Part print with two shaded views. Sizes in mm from the minimum x, y, z corner. Coordinates: 2 decimals unless noted, no trailing zeros. Order: outer loops, then holes, each group sorted by start corner. A loop starts at its lowest first (then second) coordinate and runs counter-clockwise, first axis right, second up. Notation, with made-up numbers: M -12,7 L 17,7 A12 ccw 17,21 Z; hole C 37.5,-20.5 d6. An arc over 180 degrees is marked long. Answer in a Markdown table with one row per item. Add a question column.
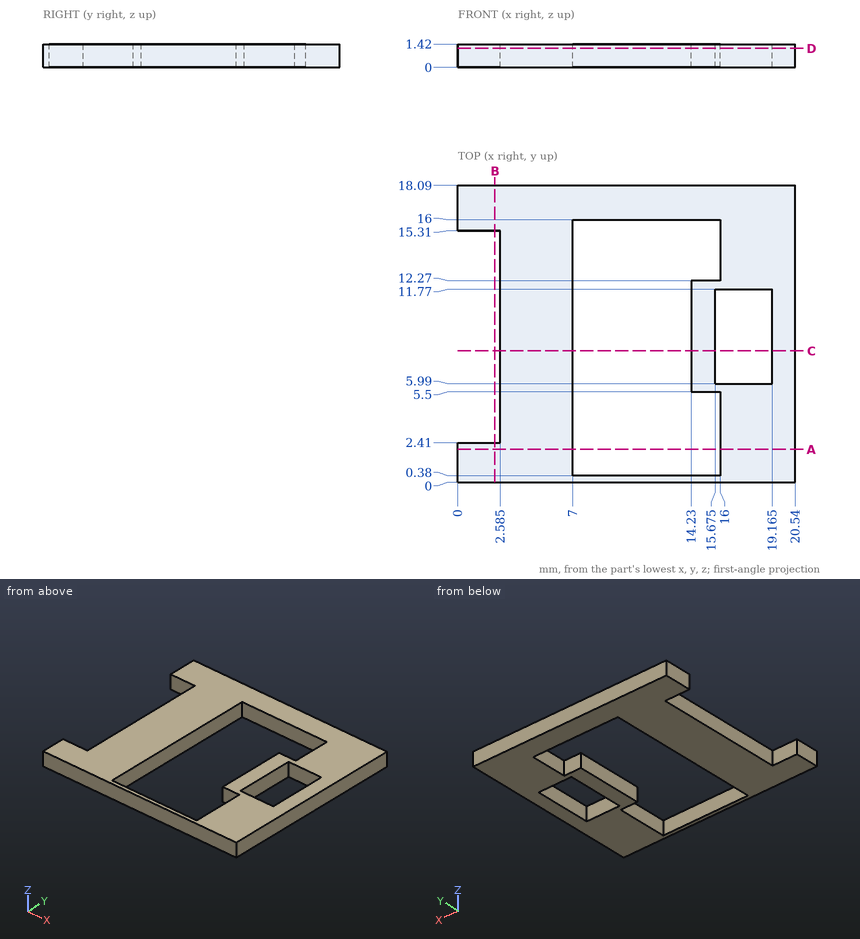
(1) Slice it at C-C (y = 8). List the corners of the cut face in (x, z) (3 decimals), and give its area (3 significant figures).
(2) Wall check: line 1 (X direction, y = 7.75, z = 1.3) (3 decimals); line 2 (X direction, y = 5, z = 0.4) (3 decimals); line 3 (X direction, y = 1.75, z = 1.05). Give the ranges that are in metal, low to high.
(3) Drop flat-ended pins along their axis: P1, Ø0.7, axis at y = 8.5, z = 1, coming from the -X side (3 decimals); P2, Ø4, axis at x = 12.5, y = 12.5, coming from the -Z side. Give the stop position or say it passes through.
(4) Slice it at A-A (y = 2). List the corners of the cut face in (x, z), and give its area (3 significant figures).
(5) Slice it at D-D (z = 1.15). List the corners of the cut face in (x, y) (3 decimals).
(6) Slice it at B-B (x = 2.25). List the corners of the cut face in (y, z), and give its area (3 significant figures).
Computed:
| question | item | result |
|---|---|---|
| 1 | outline | M 2.585,0 L 7,0 L 7,1.42 L 2.585,1.42 Z; M 14.23,0 L 15.675,0 L 15.675,1.42 L 14.23,1.42 Z; M 19.165,0 L 20.54,0 L 20.54,1.42 L 19.165,1.42 Z |
| 1 | area | 10.3 mm^2 |
| 2 | line 1 | x = 2.585 to 7, 14.23 to 15.675, 19.165 to 20.54 |
| 2 | line 2 | x = 2.585 to 7, 16 to 20.54 |
| 2 | line 3 | x = 0 to 7, 16 to 20.54 |
| 3 | P1 | stops at x = 2.585 |
| 3 | P2 | stops at z = 0 |
| 4 | outline | M 0,0 L 7,0 L 7,1.42 L 0,1.42 Z; M 16,0 L 20.54,0 L 20.54,1.42 L 16,1.42 Z |
| 4 | area | 16.4 mm^2 |
| 5 | outline | M 0,0 L 20.54,0 L 20.54,18.09 L 0,18.09 L 0,15.31 L 2.585,15.31 L 2.585,2.41 L 0,2.41 Z; hole M 7,0.38 L 16,0.38 L 16,5.5 L 14.23,5.5 L 14.23,12.27 L 16,12.27 L 16,16 L 7,16 Z; hole M 15.675,5.99 L 19.165,5.99 L 19.165,11.77 L 15.675,11.77 Z |
| 6 | outline | M 0,0 L 2.41,0 L 2.41,1.42 L 0,1.42 Z; M 15.31,0 L 18.09,0 L 18.09,1.42 L 15.31,1.42 Z |
| 6 | area | 7.37 mm^2 |
